Read the model definition and answer for the solid it produces. Units are mm, in the model's axes. Face numbers are marked on the shaded views. A direction names the side the tool comes from. Give positions to 0.01 mm unless a question says otherwise; leave off trailing zeros. Order: outer loops, then holes, each group sorted by start corner. A loop starts at its lowest first (then second) coordinate and runs counter-clockwise, first axis right, second up. Notation, with made-up numbers: (-14, 40) - (-2, 40) arc R8 cw to (-2, 44) - close; hole circle Ø11 at (22, 19). An arc over 180 degrees is marked (long way). Return JSON: item names as keys, results as strings.
```python
from build123d import *

# Parameters (mm, degrees)
F0_W     = 57.15
F0_H     = 25.4
F1_DEPTH = 44.45
F3_DEPTH = 12.7
F4_R     = 12.7
F5_DEPTH = 25.4


with BuildPart() as f1:
    # F0 (on Top) → F1 (new body)
    with BuildSketch(Plane.XY):
        with Locations((28.575, 12.7)):
            Rectangle(F0_W, F0_H)
    extrude(amount=F1_DEPTH)

    # F2 (on face) → F3 (cut)
    with BuildSketch(Plane.XZ):
        Polygon((57.15, 44.45), (19.05, 44.45), (44.45, 0), (57.15, 0), align=None)
    extrude(amount=-F3_DEPTH, mode=Mode.SUBTRACT)

    # F4 (on face) → F5 (cut)
    with BuildSketch(Plane(origin=(0, 25.4, 0), x_dir=(-1, 0, 0), z_dir=(0, 1, 0))):
        with Locations((-25.4, 22.439942)):
            Circle(F4_R)
    extrude(amount=-F5_DEPTH, mode=Mode.SUBTRACT)


solid = f1.part
```
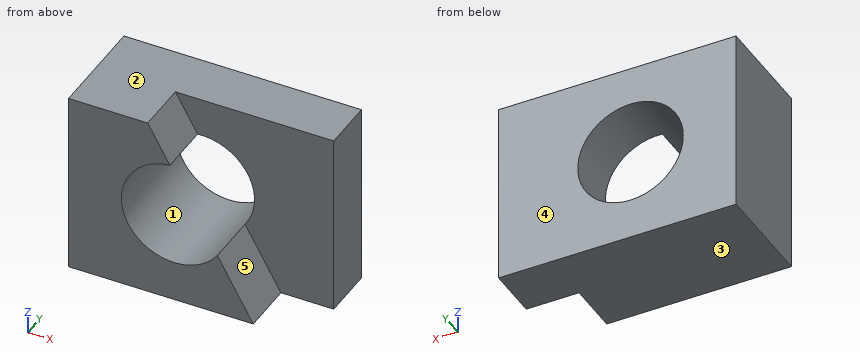
Q1. Determine the mould class of the marked faces 1, 2 and 3 for opening direction Z: released by +Z, released by -Z, zero draft, split by the parting line, or undercut.
Values:
{"face 1": "undercut", "face 2": "released by +Z", "face 3": "released by -Z"}
Q2. A cutting plane is placed at C-C (y = 3.25). Write down the section's boundary in (x, z), and give its area (3 significant figures).
Values:
{"outline": "(0, 0) - (44.45, 0) - (35.8, 15.14) arc R12.7 cw (long way) to (24.39, 35.1) - (19.05, 44.45) - (0, 44.45) - close", "area": "1,020 mm²"}
Q3. A cutting plane is placed at A-A (x = 25.4). Write down the section's boundary in (y, z).
Values:
{"outline": "(0, 0) - (25.4, 0) - (25.4, 9.74) - (0, 9.74) - close; (12.7, 35.14) - (25.4, 35.14) - (25.4, 44.45) - (12.7, 44.45) - close"}
Q4. Consider L1, parallel to Z at x = 25.4, y = 17.25; L2, parallel to Y at x = 46.5, z = 15.5; L3, parallel to Z at x = 34, y = 16 (3 decimals). Determine where each line is inside the solid, lowest interval first.
Values:
{"L1": "z = 0 to 9.74, 35.14 to 44.45", "L2": "y = 12.7 to 25.4", "L3": "z = 0 to 13.095, 31.785 to 44.45"}
Q5. Given pin 1 (1.5 mm diameter, centred on x = 22, y = 4.5, fed in from +Z); pin 2 (6 mm diameter, centred on x = 44, z = 35, fed in from -Y), each flat-ended and moving along its own axis, determine where each tip first touches the part or whether it passes through.
Values:
{"pin 1": "stops at z = 40.6", "pin 2": "stops at y = 12.7"}
Q6. A cutting plane is placed at B-B (z = 26). Write down the section's boundary in (x, y), and give its area (3 significant figures).
Values:
{"outline": "(0, 0) - (13.21, 0) - (13.21, 25.4) - (0, 25.4) - close; (37.59, 12.7) - (57.15, 12.7) - (57.15, 25.4) - (37.59, 25.4) - close", "area": "584 mm²"}
Q7. A cutting plane is placed at D-D (z = 12). Write down the section's boundary in (x, y).
Values:
{"outline": "(0, 0) - (18.17, 0) - (18.17, 25.4) - (0, 25.4) - close; (32.63, 0) - (37.59, 0) - (37.59, 12.7) - (57.15, 12.7) - (57.15, 25.4) - (32.63, 25.4) - close"}
Q8. For the marked faces 4 and 5, determine the directions among +Z, -Z, +X, -X, +Y, -Y from which every point of the face is accessible in a straight line to the end or side of a thin tool.
Values:
{"face 4": "+Z, -Z, +X, -X, +Y", "face 5": "+Z, +X, -Y"}
